For this review, take the finished solid that the model builds, in its own axes (mm). Face numbers are marked on the shaded views. A direction names the side the tool comes from. Round coordinates to 2 decimals unless told otherwise and drop trailing zeros. Loops run counter-clockwise (first coordinate to the right, second up) from the corner with the lowest first, then second, coordinate; pieces in that order, holes last.
1. Consider section A-A on x = 75. State the section outline as (y, z) points.
2. Clearance check with flat-ended pins moving along their axes: pin 1 Ø1 at (x, z) = (8.5, 86.5) entering from +Y; pin 2 Ø22.5 at (x, z) = (-73.5, 119.5) entering from +Y; pin 3 Ø24 at (x, y) = (69, -86.5) entering from +Z; pin 4 Ø12 at (x, y) = (75, -82.5) entering from +Z. State where each tip first meets the part, or that it passes through.
3. Consider section D-D on y = -5.5. State the section outline as (x, z) points.
4. Consider section C-C on x = -92. State the section outline as (y, z) points.
5. Tool access review of the marked faces 4, 5, 6 and 7: name each direction out of +Z, -Z, +X, -X, +Y, -Y from which nothing blocks a thin tool from reaching the whole face with its end or side.
6. To check wall thickness, follow line 1 along Y through (x, z) = (75, 28); line 2 along X through (y, z) = (-82, 29); line 3 along X through (y, z) = (-82, 16). State the ranges of each line that lie inside material, in increasing order.
7. Consider section B-B on y = 56. State the section outline as (x, z) points.
8. Draft analysis for pull direction Y (two halves, no side actions). For the marked faces 1, 2 and 3, state which applies: released by +Y, released by -Y, zero draft, split by the parting line, or undercut.
from build123d import *

# Parameters (mm, degrees)
F0_W            = 210
F0_H            = 225
F1_DEPTH        = 25
F3_DEPTH        = 95
F5_DEPTH        = 10
F5_DEPTH_BACK   = 127
F7_DEPTH        = 10
F7_DEPTH_BACK   = 127
F8_W            = 60
F8_H            = 60
F9_DEPTH        = 10
F10_R           = 10
F12_DEPTH       = 20
F14_D           = 15
F14_CBORE_D     = 30
F14_CBORE_DEPTH = 10
F15_R           = 10
F16_R           = 19.5
F17_DEPTH       = 235.001
F18_R           = 19.5
F19_DEPTH       = 137.0010001
F20_SIZE        = 2


with BuildPart() as f1:
    # F0 (on Top) → F1 (new body)
    with BuildSketch(Plane.XY):
        Rectangle(F0_W, F0_H)
    extrude(amount=F1_DEPTH)

    # F2 (on face) → F3 (join)
    with BuildSketch(Plane.XY.offset(25)):
        with BuildLine():
            Line((-71, -32.5), (-71, -112.5))
            Line((-71, -112.5), (-56, -112.5))
            Line((-56, -112.5), (-56, -46.4818166789))
            ThreePointArc((-56, -46.4818166789), (7.4888527117, -14.9888527117), (38.9818166789, 48.5))
            Line((38.9818166789, 48.5), (105, 48.5))
            Line((105, 48.5), (105, 63.5))
            Line((105, 63.5), (25, 63.5))
            ThreePointArc((25, 63.5), (-3.1177490061, -4.3822509939), (-71, -32.5))
        make_face()
    extrude(amount=F3_DEPTH)

    # F4 (on face) → F5 (join, two sides)
    with BuildSketch(Plane.XZ.offset(112.5)) as f5_sk:
        with BuildLine():
            ThreePointArc((-56, 83.2576538583), (-34.4526249034, 96.2829175487), (-26, 120))
            ThreePointArc((-26, 120), (-87.2170824513, 149.0473750966), (-71, 83.2576538583))
            Line((-71, 83.2576538583), (-71, 120))
            Line((-71, 120), (-56, 120))
            Line((-56, 120), (-56, 83.2576538583))
        make_face()
        with BuildLine():
            Line((-71, 120), (-71, 83.2576538583))
            ThreePointArc((-71, 83.2576538583), (-63.5, 82.5), (-56, 83.2576538583))
            Line((-56, 83.2576538583), (-56, 120))
            Line((-56, 120), (-71, 120))
        make_face()
    extrude(amount=F5_DEPTH)
    extrude(f5_sk.sketch, amount=-F5_DEPTH_BACK)

    # F6 (on face) → F7 (join, two sides)
    with BuildSketch(Plane.YZ.offset(105)) as f7_sk:
        with BuildLine():
            ThreePointArc((63.5, 80.7094158862), (86.8220700148, 94.504902432), (96, 120))
            ThreePointArc((96, 120), (30.504902432, 150.8220700148), (48.5, 80.7094158862))
            Line((48.5, 80.7094158862), (48.5, 120))
            Line((48.5, 120), (63.5, 120))
            Line((63.5, 120), (63.5, 80.7094158862))
        make_face()
        with BuildLine():
            Line((48.5, 120), (48.5, 80.7094158862))
            ThreePointArc((48.5, 80.7094158862), (56, 80), (63.5, 80.7094158862))
            Line((63.5, 80.7094158862), (63.5, 120))
            Line((63.5, 120), (48.5, 120))
        make_face()
    extrude(amount=F7_DEPTH)
    extrude(f7_sk.sketch, amount=-F7_DEPTH_BACK)

    # F8 (on face) → F9 (join)
    with BuildSketch(Plane.XY.offset(25)):
        with Locations((75, -82.5)):
            Rectangle(F8_W, F8_H)
    extrude(amount=F9_DEPTH)

    # F10
    f10_edges = [f1.edges().sort_by_distance(p)[0] for p in [
        (45, -52.5, 30),
    ]]
    fillet(f10_edges, radius=F10_R)

    # F11 (on face) → F12 (cut)
    with BuildSketch(Plane.XY.offset(25)):
        with BuildLine():
            ThreePointArc((46.5755076536, 39.5), (13.8528137424, -21.3528137424), (-47, -54.0755076536))
            Line((-47, -54.0755076536), (-47, -103.5))
            Line((-47, -103.5), (36, -103.5))
            Line((36, -103.5), (36, -62.5))
            ThreePointArc((36, -62.5), (41.5649711575, -49.0649711575), (55, -43.5))
            Line((55, -43.5), (96, -43.5))
            Line((96, -43.5), (96, 39.5))
            Line((96, 39.5), (46.5755076536, 39.5))
        make_face()
    extrude(amount=-F12_DEPTH, mode=Mode.SUBTRACT)

    # F14 (through all)
    with Locations(Plane.XY.offset(35)):
        with Locations((75, -82.5)):
            CounterBoreHole(F14_D / 2, F14_CBORE_D / 2, F14_CBORE_DEPTH)

    # F15
    f15_edges = [f1.edges().sort_by_distance(p)[0] for p in [
        (-47, -54.075508, 15),
        (-47, -103.5, 15),
        (36, -103.5, 15),
        (46.575508, 39.5, 15),
        (96, 39.5, 15),
        (96, -43.5, 15),
    ]]
    fillet(f15_edges, radius=F15_R)

    # F16 (on face) → F17 (cut, through all)
    with BuildSketch(Plane.XZ.offset(122.5)):
        with Locations((-63.5, 120)):
            Circle(F16_R)
    extrude(amount=-F17_DEPTH, mode=Mode.SUBTRACT)

    # F18 (on face) → F19 (cut, through all)
    with BuildSketch(Plane(origin=(-22, 0, 0), x_dir=(0, -1, 0), z_dir=(-1, 0, 0))):
        with Locations((-56, 120)):
            Circle(F18_R)
    extrude(amount=-F19_DEPTH, mode=Mode.SUBTRACT)

    # F20
    f20_edges = [f1.edges().sort_by_distance(p)[0] for p in [
        (-22, 75.5, 120),
        (-83, 14.5, 120),
        (-83, -122.5, 120),
        (115, 75.5, 120),
    ]]
    chamfer(f20_edges, length=F20_SIZE)


solid = f1.part
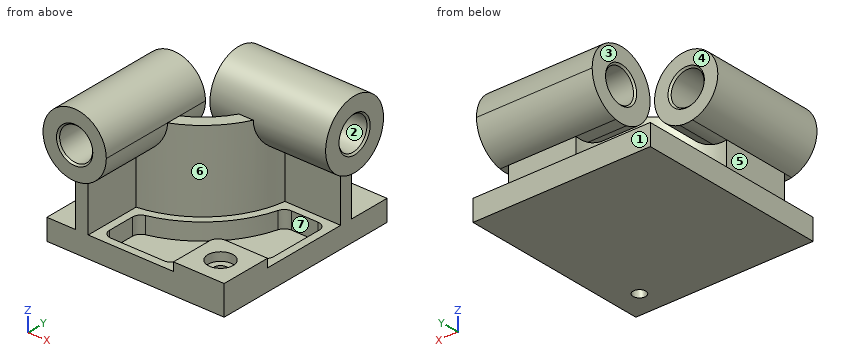
Resolved:
1. outline: (-112.5, 0) - (-90, 0) - (-90, 25) - (-97.5, 25) - (-97.5, 35) - (-112.5, 35) - close; (-75, 0) - (112.5, 0) - (112.5, 25) - (63.5, 25) - (63.5, 80.71) arc R40 ccw (long way) to (48.5, 80.71) - (48.5, 25) - (39.5, 25) - (39.5, 5) - (-43.5, 5) - (-43.5, 25) - (-52.5, 25) - (-52.5, 35) - (-67.5, 35) - (-67.5, 25) - (-75, 25) - close; hole circle Ø39 at (56, 120)
2. pin 1: stops at y = 78.61
2. pin 2: stops at y = 14.26
2. pin 3: stops at z = 35
2. pin 4: passes through
3. outline: (-105, 0) - (105, 0) - (105, 25) - (96, 25) - (96, 5) - (27.18, 5) - (27.18, 25) - (15.95, 25) - (15.95, 120) - (-4.25, 120) - (-4.25, 25) - (-105, 25) - close; circle Ø75 at (-63.5, 120); hole circle Ø39 at (-63.5, 120)
4. outline: (-122.5, 95.63) - (14.5, 95.63) - (14.5, 144.37) - (-122.5, 144.37) - close; (-112.5, 0) - (112.5, 0) - (112.5, 25) - (-112.5, 25) - close
5. face 4: +Z, -X, +Y
5. face 5: -X, +Y, -Y
5. face 6: +X, -Y
5. face 7: none
6. line 1: y = -112.5 to -97.5, -67.5 to -52.5, 48.5 to 63.5
6. line 2: x = -71 to -56, 45 to 60.01, 89.99 to 105
6. line 3: x = -105 to -47, 36 to 67.52, 82.48 to 105
7. outline: (-105, 0) - (105, 0) - (105, 80) - (115, 80) - (115, 98.5) - (113, 100.5) - (-20, 100.5) - (-22, 98.5) - (-22, 80) - (24.71, 80) - (24.71, 25) - (-105, 25) - close; (-22, 141.5) - (-20, 139.5) - (113, 139.5) - (115, 141.5) - (115, 160) - (-22, 160) - close
8. face 1: released by +Y
8. face 2: undercut
8. face 3: zero draft
